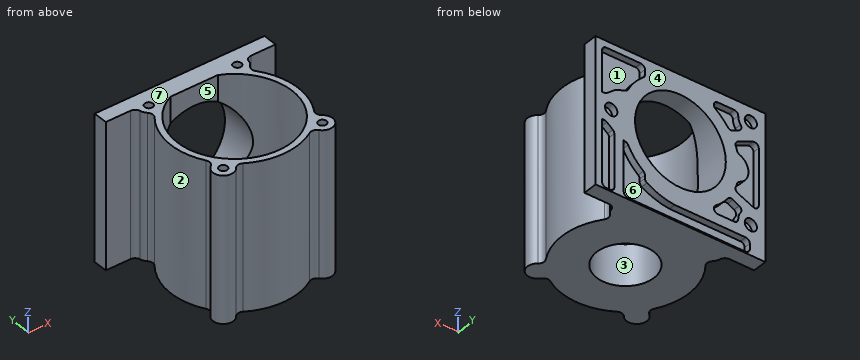
from build123d import *

# Parameters (mm, degrees)
SKETCH1_R           = 2
BOSS_EXTRUDE1_DEPTH = 71
BOSS_EXTRUDE2_START = -20
BOSS_EXTRUDE2_DEPTH = 20
SKETCH4_R           = 22.25
CUT_EXTRUDE1_DEPTH  = 20
SKETCH5_R           = 3.022127891
SKETCH5_R_2         = 2.984467426
CUT_EXTRUDE2_DEPTH  = 3.3
BOSS_EXTRUDE3_START = -53.3
SKETCH6_R           = 2
BOSS_EXTRUDE3_DEPTH = 53.3
SKETCH7_R           = 22.25
CUT_EXTRUDE4_DEPTH  = 20
SKETCH8_R           = 14
CUT_EXTRUDE5_DEPTH  = 29


with BuildPart() as part:
    # Sketch1 → Boss-Extrude1 (new body)
    with BuildSketch(Plane.XY):
        with BuildLine():
            Line((-41.6, 34.7), (41.6, 34.7))
            Line((41.6, 34.7), (41.6, 27.7))
            Line((41.6, 27.7), (29.558116823, 27.7))
            ThreePointArc((29.558116823, 27.7), (27.645984505, 27.011655251), (26.611323014, 25.2625))
            ThreePointArc((26.611323014, 25.2625), (26.087125484, 23.80143168), (25.140096153, 22.571537728))
            ThreePointArc((25.140096153, 22.571537728), (24.214825318, 20.64727444), (24.803787329, 18.594949156))
            ThreePointArc((24.803787329, 18.594949156), (30.963546179, 1.502933138), (26.488095667, -16.1053031))
            ThreePointArc((26.488095667, -16.1053031), (26.107899632, -18.243064514), (27.269662352, -20.077425512))
            ThreePointArc((27.269662352, -20.077425512), (27.850113241, -27.620894202), (20.302105128, -27.102804788))
            ThreePointArc((20.302105128, -27.102804788), (18.458205593, -25.956241491), (16.323659246, -26.35409169))
            ThreePointArc((16.323659246, -26.35409169), (0, -31), (-16.323659246, -26.35409169))
            ThreePointArc((-16.323659246, -26.35409169), (-18.458205593, -25.956241491), (-20.302105128, -27.102804788))
            ThreePointArc((-20.302105128, -27.102804788), (-27.850113241, -27.620894202), (-27.269662352, -20.077425512))
            ThreePointArc((-27.269662352, -20.077425512), (-26.107899632, -18.243064514), (-26.488095667, -16.1053031))
            ThreePointArc((-26.488095667, -16.1053031), (-30.963546179, 1.502933138), (-24.803787329, 18.594949156))
            ThreePointArc((-24.803787329, 18.594949156), (-24.214825318, 20.64727444), (-25.140096153, 22.571537728))
            ThreePointArc((-25.140096153, 22.571537728), (-26.087125484, 23.80143168), (-26.611323014, 25.2625))
            ThreePointArc((-26.611323014, 25.2625), (-27.645984505, 27.011655251), (-29.558116823, 27.7))
            Line((-29.558116823, 27.7), (-41.6, 27.7))
            Line((-41.6, 27.7), (-41.6, 34.7))
        make_face()
        with Locations((-24.3, -24.1)):
            Circle(SKETCH1_R, mode=Mode.SUBTRACT)
        with Locations(Location((24.3, -24.1, 0), (0, 0, 180))):
            Circle(SKETCH1_R, mode=Mode.SUBTRACT)
        with Locations((-21.7, 26.2)):
            Circle(SKETCH1_R, mode=Mode.SUBTRACT)
        with Locations(Location((21.7, 26.2, 0), (0, 0, 180))):
            Circle(SKETCH1_R, mode=Mode.SUBTRACT)
        with BuildLine():
            Line((0, 25.5), (-11.565033506, 25.5))
            ThreePointArc((-11.565033506, 25.5), (0, -28), (11.565033506, 25.5))
            Line((11.565033506, 25.5), (0, 25.5))
        make_face(mode=Mode.SUBTRACT)
    extrude(amount=-BOSS_EXTRUDE1_DEPTH)

    # Sketch3 → Boss-Extrude2 (add)
    with BuildSketch(Plane(origin=(0, 0, -71), x_dir=(-1, 0, 0), z_dir=(0, 0, -1)).offset(BOSS_EXTRUDE2_START)):
        with BuildLine():
            Line((-11.565033506, 25.5), (11.565033506, 25.5))
            ThreePointArc((11.565033506, 25.5), (0, -28), (-11.565033506, 25.5))
        make_face()
    extrude(amount=BOSS_EXTRUDE2_DEPTH)

    # Sketch4 → Cut-Extrude1 (cut)
    with BuildSketch(Plane(origin=(0, 34.7, 0), x_dir=(1, 0, 0), z_dir=(0, 1, 0))):
        with Locations(Location((0, 31.75, 0), (0, 0, 180))):
            Circle(SKETCH4_R)
    extrude(amount=-CUT_EXTRUDE1_DEPTH, mode=Mode.SUBTRACT)

    # Sketch5 → Cut-Extrude2 (cut)
    with BuildSketch(Plane(origin=(0, 34.7, 0), x_dir=(1, 0, 0), z_dir=(0, 1, 0))):
        with Locations(Location((33.927872109, 31.75, 0), (0, 0, 180))):
            Circle(SKETCH5_R)
        with Locations(Location((-34.5, 7.1, 0), (0, 0, 180))):
            Circle(SKETCH5_R_2)
        with Locations((-34.5, 56.4)):
            Circle(SKETCH5_R_2)
        with BuildLine():
            Line((17.4, 5.222938284), (17.4, 7.752337891))
            ThreePointArc((17.4, 7.752337891), (17.597173424, 8.623464734), (18.150257171, 9.324776153))
            ThreePointArc((18.150257171, 9.324776153), (22.362877615, 13.522981462), (25.625145816, 18.495777959))
            ThreePointArc((25.625145816, 18.495777959), (26.071081355, 19.072193711), (26.692339737, 19.453181438))
            Line((26.692339737, 19.453181438), (31.637345031, 21.365422694))
            ThreePointArc((31.637345031, 21.365422694), (31.920318143, 21.500934926), (32.178933924, 21.67857283))
            Line((32.178933924, 21.67857283), (36.043799869, 24.800690212))
            ThreePointArc((36.043799869, 24.800690212), (36.640870302, 25.134367752), (37.315009001, 25.25))
            Line((37.315009001, 25.25), (38.4, 25.25))
            Line((38.4, 25.25), (38.4, 5.222938284))
            ThreePointArc((38.4, 5.222938284), (37.807495095, 3.792504905), (36.377061716, 3.2))
            Line((36.377061716, 3.2), (19.422938284, 3.2))
            ThreePointArc((19.422938284, 3.2), (17.992504905, 3.792504905), (17.4, 5.222938284))
        make_face()
        with BuildLine():
            Line((38.4, 38.25), (37.315009001, 38.25))
            ThreePointArc((37.315009001, 38.25), (36.640870302, 38.365632248), (36.043799869, 38.699309788))
            Line((36.043799869, 38.699309788), (33.151729153, 41.035583382))
            ThreePointArc((33.151729153, 41.035583382), (32.597581207, 41.737230892), (32.4, 42.609211879))
            Line((32.4, 42.609211879), (32.4, 68.330496056))
            ThreePointArc((32.4, 68.330496056), (32.992504905, 69.760929435), (34.422938284, 70.35343434))
            Line((34.422938284, 70.35343434), (36.377061716, 70.35343434))
            ThreePointArc((36.377061716, 70.35343434), (37.807495095, 69.760929435), (38.4, 68.330496056))
            Line((38.4, 68.330496056), (38.4, 38.25))
        make_face()
        with BuildLine():
            Line((27.8, 43.618484612), (26.692339737, 44.046818562))
            ThreePointArc((26.692339737, 44.046818562), (26.071081355, 44.427806289), (25.625145816, 45.004222041))
            ThreePointArc((25.625145816, 45.004222041), (22.362877615, 49.977018538), (18.150257171, 54.175223847))
            ThreePointArc((18.150257171, 54.175223847), (17.597173424, 54.876535266), (17.4, 55.747662109))
            Line((17.4, 55.747662109), (17.4, 57.336521607))
            ThreePointArc((17.4, 57.336521607), (17.137782315, 58.332584995), (16.41910772, 59.070424553))
            ThreePointArc((16.41910772, 59.070424553), (9.869306341, 62.058241262), (2.816060384, 63.5))
            Line((2.816060384, 63.5), (-31.977061716, 63.5))
            ThreePointArc((-31.977061716, 63.5), (-33.407495095, 64.092504905), (-34, 65.522938284))
            Line((-34, 65.522938284), (-34, 68.330496056))
            ThreePointArc((-34, 68.330496056), (-33.407495095, 69.760929435), (-31.977061716, 70.35343434))
            Line((-31.977061716, 70.35343434), (25.777061716, 70.35343434))
            ThreePointArc((25.777061716, 70.35343434), (27.207495095, 69.760929435), (27.8, 68.330496056))
            Line((27.8, 68.330496056), (27.8, 43.618484612))
        make_face()
        with BuildLine():
            Line((-35.596515067, 47.366259615), (-28.191539915, 44.117682775))
            ThreePointArc((-28.191539915, 44.117682775), (-27.15636094, 43.073143107), (-27.115282556, 41.603118892))
            ThreePointArc((-27.115282556, 41.603118892), (-27.46160788, 40.592092097), (-27.77025027, 39.568932147))
            ThreePointArc((-27.77025027, 39.568932147), (-28.20915438, 38.772659729), (-28.955222822, 38.252978614))
            ThreePointArc((-28.955222822, 38.252978614), (-33.364611091, 31.75), (-28.955222822, 25.247021386))
            ThreePointArc((-28.955222822, 25.247021386), (-28.20915438, 24.727340271), (-27.77025027, 23.931067853))
            ThreePointArc((-27.77025027, 23.931067853), (-27.46160788, 22.907907903), (-27.115282556, 21.896881108))
            ThreePointArc((-27.115282556, 21.896881108), (-27.15636094, 20.426856893), (-28.191539915, 19.382317225))
            Line((-28.191539915, 19.382317225), (-35.596515067, 16.133740385))
            ThreePointArc((-35.596515067, 16.133740385), (-37.493853311, 16.290884715), (-38.4, 17.965245767))
            Line((-38.4, 17.965245767), (-38.4, 45.534754233))
            ThreePointArc((-38.4, 45.534754233), (-37.493853311, 47.209115285), (-35.596515067, 47.366259615))
        make_face()
        with BuildLine():
            Line((-18.369728815, 5.007277506), (-26.334797191, 5.007277506))
            ThreePointArc((-26.334797191, 5.007277506), (-27.757017341, 5.60111612), (-28.334668249, 7.029987663))
            ThreePointArc((-28.334668249, 7.029987663), (-28.624699957, 8.970044578), (-29.509419908, 10.720818646))
            ThreePointArc((-29.509419908, 10.720818646), (-29.837700915, 12.352292131), (-28.817875571, 13.667370236))
            Line((-28.817875571, 13.667370236), (-25.756437816, 15.269338838))
            ThreePointArc((-25.756437816, 15.269338838), (-24.378292278, 15.445800084), (-23.217742786, 14.681896575))
            ThreePointArc((-23.217742786, 14.681896575), (-20.424298577, 11.421897229), (-17.177523303, 8.613093816))
            ThreePointArc((-17.177523303, 8.613093816), (-16.470830105, 6.379437009), (-18.369728815, 5.007277506))
        make_face()
        with BuildLine():
            Line((-18.369728815, 58.492722494), (-26.334797191, 58.492722494))
            ThreePointArc((-26.334797191, 58.492722494), (-27.757017341, 57.89888388), (-28.334668249, 56.470012337))
            ThreePointArc((-28.334668249, 56.470012337), (-28.624699957, 54.529955422), (-29.509419908, 52.779181354))
            ThreePointArc((-29.509419908, 52.779181354), (-29.837700915, 51.147707869), (-28.817875571, 49.832629764))
            Line((-28.817875571, 49.832629764), (-25.756437816, 48.230661162))
            ThreePointArc((-25.756437816, 48.230661162), (-24.378292278, 48.054199916), (-23.217742786, 48.818103425))
            ThreePointArc((-23.217742786, 48.818103425), (-20.424298577, 52.078102771), (-17.177523303, 54.886906184))
            ThreePointArc((-17.177523303, 54.886906184), (-16.470830105, 57.120562991), (-18.369728815, 58.492722494))
        make_face()
    extrude(amount=-CUT_EXTRUDE2_DEPTH, mode=Mode.SUBTRACT)

    # Sketch6 → Boss-Extrude3 (add)
    with BuildSketch(Plane(origin=(0, 0, -71), x_dir=(-1, 0, 0), z_dir=(0, 0, -1)).offset(BOSS_EXTRUDE3_START)):
        with Locations((-21.7, 26.2)):
            Circle(SKETCH6_R)
        with Locations(Location((21.7, 26.2, 0), (0, 0, 180))):
            Circle(SKETCH6_R)
        with Locations(Location((24.3, -24.1, 0), (0, 0, 180))):
            Circle(SKETCH6_R)
        with Locations((-24.3, -24.1)):
            Circle(SKETCH6_R)
    extrude(amount=BOSS_EXTRUDE3_DEPTH)

    # Sketch7 → Cut-Extrude4 (cut)
    with BuildSketch(Plane(origin=(0, 34.7, 0), x_dir=(1, 0, 0), z_dir=(0, 1, 0))):
        with Locations(Location((0, 31.75, 0), (0, 0, 180))):
            Circle(SKETCH7_R)
    extrude(amount=-CUT_EXTRUDE4_DEPTH, mode=Mode.SUBTRACT)

    # Sketch8 → Cut-Extrude5 (cut)
    with BuildSketch(Plane.XY.offset(-51)):
        Circle(SKETCH8_R)
    extrude(amount=-CUT_EXTRUDE5_DEPTH, mode=Mode.SUBTRACT)


solid = part.part
Read the model definition and answer for the solid it produces. Units are mm, in the model's axes. Face numbers are marked on the shaded views. A direction names the side the tool comes from. Round coordinates to 2 decimals unless told otherwise and drop trailing zeros. Write each loop counter-clockwise with the first axis right and the second up, starting at its lowest first coordinate (ties: lowest second). Pieces come first, ordered by that corner, then holes.
Q1. Find section C-C on y = -24.1. Determine the outline of the cut face in (x, z).
Values:
outline: (-29.3, -71) - (29.3, -71) - (29.3, 0) - (26.3, 0) - (26.3, -17.7) - (22.3, -17.7) - (22.3, 0) - (14.25, 0) - (14.25, -51) - (-14.25, -51) - (-14.25, 0) - (-22.3, 0) - (-22.3, -17.7) - (-26.3, -17.7) - (-26.3, 0) - (-29.3, 0) - close
Q2. Find section A-A on x = 1. Determine the outline of the cut face in (y, z), and give its area (3 significant figures).
Values:
outline: (-30.98, -71) - (-13.96, -71) - (-13.96, -51) - (-27.98, -51) - (-27.98, 0) - (-30.98, 0) - close; (13.96, -71) - (34.7, -71) - (34.7, -70.35) - (31.4, -70.35) - (31.4, -63.5) - (34.7, -63.5) - (34.7, -53.98) - (14.7, -53.98) - (14.7, -51) - (13.96, -51) - close; (25.5, -9.52) - (34.7, -9.52) - (34.7, 0) - (25.5, 0) - close
area: 914 mm2
Q3. A tool of negligible diameter and unlimited length cuts with its end or side. For the marked faces 5, 6 and 7, from which of +Z, -Z, +X, -X, +Y, -Y can it reach the whole face along a straight path? Write none if from no direction.
Values:
face 5: +Z
face 6: +Y
face 7: +Z, +X, -X, +Y, -Y
Q4. Straight lines are drawn through the part: line 1 (Y direction, x = 24, z = -8); line 2 (Y direction, x = 21.7, z = -11.25); line 3 (X direction, y = 26.2, z = -5.5). For each, find the intervals that lie inside material, in ascending order.
Values:
line 1: y = -29.09 to -26.08, -22.12 to -14.42, 14.42 to 31.4
line 2: y = -28.37 to -17.69, 17.69 to 24.2, 28.2 to 31.4
line 3: x = -26.96 to -23.7, -19.7 to 19.7, 23.7 to 26.96
Q5. The mould has two halves that part along X. Classify the marked faces 1, 2, 3 and 4: released by +X, released by -X, zero draft, split by the parting line, or undercut.
Values:
face 1: undercut
face 2: released by -X
face 3: undercut
face 4: zero draft
Q6. Flat-ended cylindrical pins translate along their axes: P1, Ø1, axis at x = 23, z = -36.5, coming from the -Y side; P2, Ø2, axis at x = 1, z = -25.5, coming from the -Y side; P3, Ø2, axis at y = 22.5, z = -18, coming from the +X side. Find the tip coordinate at first contact, or state that the pin passes through.
Values:
P1: stops at y = -29.04
P2: stops at y = -31
P3: stops at x = 25.91
